Autodesk Fusion 360 part; units mm, degrees
sketch "Sketch1" plane through (0, 0, 0) normal (0, 0, 1) x (1, 0, 0)
  line L0 (0, 0) -> (-40, 0)
  line L1 (-40, 0) -> (-40, -10)
  line L2 (-40, -10) -> (0, -10)
  line L3 (0, -10) -> (0, 0)
  dimension "SideLenght" = 40
  dimension "SideWidth" = 10
extrude "Extrude5" add sketch "Sketch1" along normal blind 10
sketch "Sketch5" plane through (0, 0, 0) normal (1, 0, 0) x (0, 1, 0)
  line L0 (-10, 0) -> (0, 0)
  line L1 (0, 0) -> (0, 10)
  line L2 (0, 10) -> (-10, 10)
  line L3 (-10, 10) -> (-10, 0)
  line L4 (-10, 10) -> (-7.9, 10) construction
  line L5 (-7.9, 10) -> (-7.9, 7.9) construction
  line L6 (0, 0) -> (-2.1, 0) construction
  line L7 (-2.1, 0) -> (-2.1, 2.1) construction
  line L8 (-7.9, 7.9) -> (-2.1, 7.9)
  line L9 (-2.1, 7.9) -> (-2.1, 2.1)
  line L10 (-2.1, 2.1) -> (-7.9, 2.1)
  line L11 (-7.9, 2.1) -> (-7.9, 7.9)
  dimension "PegOffset" = 2.1
  dimension "d15" = 2.1
  dimension "d16" = 2.1
  dimension "d17" = 2.1
sketch "Sketch6" plane through (-40, 0, 0) normal (-1, 0, 0) x (0, -1, 0)
  line L0 (0, 0) -> (10, 0)
  line L1 (10, 0) -> (10, 10)
  line L2 (10, 10) -> (0, 10)
  line L3 (0, 10) -> (0, 0)
  line L4 (0, 10) -> (2.1, 10) construction
  line L5 (2.1, 10) -> (2.1, 7.9) construction
  line L6 (10, 0) -> (7.9, 0) construction
  line L7 (7.9, 0) -> (7.9, 2.1) construction
  line L8 (2.1, 7.9) -> (7.9, 7.9)
  line L9 (7.9, 7.9) -> (7.9, 2.1)
  line L10 (7.9, 2.1) -> (2.1, 2.1)
  line L11 (2.1, 2.1) -> (2.1, 7.9)
  dimension "d18" = 2.1
  dimension "d19" = 2.1
  dimension "d20" = 2.1
  dimension "d21" = 2.1
extrude "Extrude6" add sketch "Sketch6" along normal blind 14 contours L8 L9 L10 L11
extrude "Extrude7" add sketch "Sketch5" along normal blind 14 contours L8 L9 L10 L11
sketch "Sketch7" plane through (0, 0, 7.9) normal (0, 0, 1) x (-1, 0, 0)
  line L0 (40, 7.9) -> (40, 2.1)
  line L1 (40, 2.1) -> (54, 2.1)
  line L2 (54, 2.1) -> (54, 7.9)
  line L3 (54, 7.9) -> (40, 7.9)
  line L4 (40, 5) -> (54, 5) construction
  line L5 (40, 5) -> (50, 5) construction
  circle A0 centre (45, 5) radius 1.6
  dimension "d31" = 3.2
  dimension "d33" = 10
sketch "Sketch8" plane through (0, 0, 7.9) normal (0, 0, 1) x (-1, 0, 0)
  line L0 (0, 2.1) -> (0, 7.9)
  line L1 (0, 7.9) -> (-14, 7.9)
  line L2 (-14, 7.9) -> (-14, 2.1)
  line L3 (-14, 2.1) -> (0, 2.1)
  line L4 (0, 5) -> (-14, 5) construction
  line L5 (-10, 5) -> (0, 5) construction
  circle A0 centre (-5, 5) radius 1.6
  dimension "d32" = 3.2
  dimension "d34" = 10
extrude "Extrude8" cut sketch "Sketch8" sketch "Sketch7" against normal blind 11 contours A0 of sketch 2 contours A0
fillet "Fillet1" radius 1 1 edges at (-20, 0, 0)
fillet "Fillet1" radius 1 3 edges at (-20, 0, 10) (-20, -10, 10) (-20, -10, 0)
sketch "Sketch9" plane through (0, 0, 10) normal (0, 0, 1) x (-1, 0, 0)
  line L0 (40, 9) -> (0, 9)
  line L1 (0, 9) -> (0, 1)
  line L2 (0, 1) -> (40, 1)
  line L3 (40, 1) -> (40, 9)
  line L4 (20, 1) -> (20, 9) construction
  line L5 (20, 9) -> (40, 9) construction
  line L6 (10, 1) -> (0, 1)
  circle A0 centre (4, 5) radius 4 construction
  line L7 (40, 5) -> (0, 5) construction
  circle A1 centre (12, 5) radius 4 construction
  circle A2 centre (20, 5) radius 4 construction
  circle A3 centre (28, 5) radius 4 construction
  circle A4 centre (4, 5) radius 3.05
  circle A5 centre (12, 5) radius 3.05
  circle A6 centre (36, 5) radius 4 construction
  circle A7 centre (20, 5) radius 3.05
  circle A8 centre (28, 5) radius 3.05
  circle A9 centre (36, 5) radius 3.05
  circle A10 centre (28, 5) radius 3.875
  circle A11 centre (36, 5) radius 3.875
  circle A12 centre (20, 5) radius 3.875
  circle A13 centre (12, 5) radius 3.875
  circle A14 centre (4, 5) radius 3.875
  dimension "d43" = 8
  dimension "d44" = 8
  dimension "d45" = 8
  dimension "d46" = 8
  dimension "d47" = 6.1
  dimension "d48" = 6.1
  dimension "d49" = 8
  dimension "d50" = 6.1
  dimension "d51" = 6.1
  dimension "d52" = 6.1
  dimension "d55" = 7.75
  dimension "d57" = 7.75
  dimension "d58" = 7.75
  dimension "d59" = 7.75
  dimension "d60" = 7.75
extrude "Extrude9" cut sketch "Sketch9" against normal blind 19 contours A4 | A5 | A7 | A8 | A9
extrude "Extrude10" cut sketch "Sketch9" against normal blind 1 contours A10 | A11 | A12 | A13 | A14
sketch "Sketch10" plane through (0, 0, 0) normal (0, 0, -1) x (1, 0, 0)
  circle A0 centre (-20, 5) radius 3.05
  circle A1 centre (-28, 5) radius 3.05
  circle A2 centre (-4, 5) radius 3.05
  circle A3 centre (-36, 5) radius 3.05
  circle A4 centre (-12, 5) radius 3.05
  line L0 (0, 9) -> (-40, 9)
  line L1 (-40, 9) -> (-40, 1)
  line L2 (-40, 1) -> (0, 1)
  line L3 (0, 1) -> (0, 9)
  circle A5 centre (-4, 5) radius 3.875
  circle A6 centre (-12, 5) radius 3.875
  circle A7 centre (-20, 5) radius 3.875
  circle A8 centre (-28, 5) radius 3.875
  circle A9 centre (-36, 5) radius 3.875
  dimension "d63" = 7.75
  dimension "d64" = 7.75
  dimension "d65" = 7.75
  dimension "d66" = 7.75
  dimension "d67" = 7.75
extrude "Extrude11" cut sketch "Sketch10" against normal blind 1 contours A5 | A6 | A7 | A8 | A9
equation "d12 = SideWidth"
equation "d15 = PegOffset"
equation "d16 = PegOffset"
equation "d17 = PegOffset"
equation "d18 = PegOffset"
equation "d19 = PegOffset"
equation "d20 = PegOffset"
equation "d21 = PegOffset"
equation "d24 = PegLenght"
equation "d47 = PinHole"
equation "d48 = PinHole"
equation "d50 = PinHole"
equation "d51 = PinHole"
equation "d52 = PinHole"
equation "d55 = PinHoleExt"
equation "PinHoleExt = 7.75 mm"
equation "d57 = PinHoleExt"
equation "d58 = PinHoleExt"
equation "d59 = PinHoleExt"
equation "d60 = PinHoleExt"
equation "d63 = PinHoleExt"
equation "d64 = PinHoleExt"
equation "d65 = PinHoleExt"
equation "d66 = PinHoleExt"
equation "d67 = PinHoleExt"
Model file for the job. Use its own axes, mm. A direction names the side the tool comes from. Give positions to 0.01 mm unless a question says otherwise; leave off trailing zeros. Loops run counter-clockwise (first coordinate to the right, second up) from the corner with the lowest first, then second, coordinate; pieces in that order, holes last.
Item 1: Slice it at C-C (x = -4). Write the cut outline in (y, z) (3 decimals).
Check values:
outline: (-10, 1) arc R1 ccw to (-9, 0) - (-8.875, 0) - (-8.875, 1) - (-8.05, 1) - (-8.05, 9) - (-8.875, 9) - (-8.875, 10) - (-9, 10) arc R1 ccw to (-10, 9) - close; (-1.95, 1) - (-1.125, 1) - (-1.125, 0) - (-1, 0) arc R1 ccw to (0, 1) - (0, 9) arc R1 ccw to (-1, 10) - (-1.125, 10) - (-1.125, 9) - (-1.95, 9) - close
Item 2: Drill centre lines: line 1 along Y through (x, z) = (-28, 6.75); line 2 along Y through (x, z) = (5, 6.25); line 3 along X through (y, z) = (-5.75, 9.25). Where is each one in solid material? Low to high.
Check values:
line 1: y = -10 to -8.05, -1.95 to 0
line 2: y = -7.9 to -6.6, -3.4 to -2.1
line 3: x = -40 to -39.8, -32.2 to -31.8, -24.2 to -23.8, -16.2 to -15.8, -8.2 to -7.8, -0.2 to 0
Item 3: Slice it at D-D (y = -5). Give the number of separate pieces and of enclosed holes in the cut face, plus the area to 3 significant figures.
Check values:
separate pieces: 8
enclosed holes: 0
area: 204 mm2
Item 4: Slice it at B-B (z = 5.5). Write the cut outline in (x, y).
Check values:
outline: (-54, -7.9) - (-40, -7.9) - (-40, -10) - (0, -10) - (0, -7.9) - (14, -7.9) - (14, -2.1) - (0, -2.1) - (0, 0) - (-40, 0) - (-40, -2.1) - (-54, -2.1) - close; hole circle Ø3.2 at (-45, -5); hole circle Ø6.1 at (-36, -5); hole circle Ø6.1 at (-28, -5); hole circle Ø6.1 at (-20, -5); hole circle Ø6.1 at (-12, -5); hole circle Ø6.1 at (-4, -5); hole circle Ø3.2 at (5, -5)
Item 5: Which spindle directions (+Z, -Z, +X, -X, +Y, -Y) get a long thin tool onto all of the face, cutting with end or side? Do faces 1 (the face through (-22, -2, 9)), 2 (the face through (7, -5, 2.1)), 3 (the face through (-10, -2, 1)). Say none if no direction does.
Check values:
face 1: +Z
face 2: -Z, +X, +Y, -Y
face 3: -Z
Item 6: Drop flat-ended pins along their axis: P1, Ø1.7, axis at x = 7.5, y = -6, coming from the -Z side; P2, Ø4, axis at x = -35.5, y = -6, coming from the -Z side; P3, Ø1.7, axis at x = -46.5, z = 6, coming from the +Y side. Give the stop position or say it passes through.
Check values:
P1: stops at z = 2.1
P2: stops at z = 1
P3: stops at y = -2.1
Item 7: Slice it at A-A (x = 5). Write the cut outline in (y, z), plus the area to 3 significant figures.
Check values:
outline: (-7.9, 2.1) - (-6.6, 2.1) - (-6.6, 7.9) - (-7.9, 7.9) - close; (-3.4, 2.1) - (-2.1, 2.1) - (-2.1, 7.9) - (-3.4, 7.9) - close
area: 15.1 mm2
